```python
from build123d import *

# Parameters (mm, degrees)
SKETCH1_R           = 1.25
BOSS_EXTRUDE1_DEPTH = 14
CHAMFER1_SIZE       = 0.35
CHAMFER2_SIZE       = 0.4
CHAMFER2_SIZE2      = 0.5


with BuildPart() as part:
    # Sketch1 → Boss-Extrude1 (new body)
    with BuildSketch(Plane.XY):
        Circle(SKETCH1_R)
    extrude(amount=BOSS_EXTRUDE1_DEPTH)

    # Chamfer1
    chamfer1_edges = [part.edges().sort_by_distance(p)[0] for p in [
        (-1.25, 0, 14),
    ]]
    chamfer(chamfer1_edges, length=CHAMFER1_SIZE)

    # Chamfer2
    chamfer2_edges = [part.edges().sort_by_distance(p)[0] for p in [
        (-1.25, 0, 0),
    ]]
    chamfer2_side = [part.faces().sort_by_distance(p)[0] for p in [
        (0, 0, 0),
    ]]
    chamfer(chamfer2_edges, length=CHAMFER2_SIZE, length2=CHAMFER2_SIZE2, reference=chamfer2_side[0])


solid = part.part
```
Could you check a few things on this model? Use its own coordinates, in mm. Coordinates: 2 decimals unless noted, no trailing zeros. Write each loop counter-clockwise with the first axis right and the second up, starting at its lowest first coordinate (ties: lowest second). Pieces come first, ordered by that corner, then holes. Notation, with made-up numbers: (45, -8.5) -> (76, -8.5) arc R21 ccw to (76, 11.5) -> close; hole circle Ø8 at (87, 28). An arc over 180 degrees is marked (long way). Write item = value, one per line. Start each with the question number.
(1) Will this pin go through, and if not, where does the flat tip stop? pin 1 (1.5 mm diameter, centred on y = -1, z = 9.5, fed in from +X).
(2) I want a section at A-A (z = 9.25). Please give me the cut outline in (x, y).
(3) I need wall thicknesses on line 1 (X direction, y = -0.25, z = 10.5); line 2 (Z direction, x = 1.15, y = -0.2); line 3 (X direction, y = 1.1, z = 5). Which ranges of each line are inside material? Lowest first, please. Write a range as [from, to].
Result set:
q1.pin_1 = 1.22
q2.outline = circle Ø2.5 at (0, 0)
q3.line_1 = [-1.22, 1.22]
q3.line_2 = [0.4, 13.73]
q3.line_3 = [-0.59, 0.59]
